The listing builds one solid part. Answer for the finished solid, in the listing's coordinates (mm). Give positions to 0.01 mm unless a question says otherwise; leave off trailing zeros. Answer as CSV lines item,"result". Start each with the question number.
(1) This flat-tipped pin is pushed along its axis until it touches: pin 1 Ø1.8 at (x, z) = (-119, -94) entering from +Y. Where does it stop, or does it pass through?
(2) Straight lines are drawn through the part: probe 1 along X at (y, z) = (1.9, -94); probe 2 along Z at (x, y) = (119, 1.9); probe 3 along Z at (x, y) = (-83, 2.9). For each, find the intervals that lie inside material, in ascending order.
(3) Find section A-A (y = 2.5). State how many separate pieces and enclosed holes the cut face has, then the cut area to 3 significant figures.
from build123d import *

# Parameters (mm, degrees)
SKETCH1_W           = 256
SKETCH1_H           = 206
BOSS_EXTRUDE1_DEPTH = 3
SKETCH2_R           = 1.5
CUT_EXTRUDE3_DEPTH  = 4
CUT_EXTRUDE6_DEPTH  = 4


with BuildPart() as part:
    # Sketch1 → Boss-Extrude1 (new body)
    with BuildSketch(Plane(origin=(0, 0, 0), x_dir=(1, 0, 0), z_dir=(0, 1, 0))):
        Rectangle(SKETCH1_W, SKETCH1_H)
    extrude(amount=BOSS_EXTRUDE1_DEPTH)

    # Sketch2 → Cut-Extrude3 (cut)
    with BuildSketch(Plane(origin=(0, 3, 0), x_dir=(1, 0, 0), z_dir=(0, 1, 0))):
        with Locations(Location((-119, 94, 0), (0, 0, 270))):
            Circle(SKETCH2_R)
        with Locations(Location((119, 94, 0), (0, 0, 270))):
            Circle(SKETCH2_R)
        with Locations(Location((119, -94, 0), (0, 0, 270))):
            Circle(SKETCH2_R)
        with Locations(Location((-119, -94, 0), (0, 0, 270))):
            Circle(SKETCH2_R)
    extrude(amount=-CUT_EXTRUDE3_DEPTH, mode=Mode.SUBTRACT)

    # Sketch5 → Cut-Extrude6 (cut)
    with BuildSketch(Plane(origin=(0, 3, 0), x_dir=(1, 0, 0), z_dir=(0, 1, 0))):
        with BuildLine():
            Line((-45.132956232, -35.122138654), (-33.270497542, -35.122138654))
            ThreePointArc((-33.270497542, -35.122138654), (-35.068849242, -42.49810977), (-39.012684657, -48.985418992))
            Line((-39.012684657, -48.985418992), (-47.527093129, -40.770618345))
            ThreePointArc((-47.527093129, -40.770618345), (-45.993141349, -38.089168216), (-45.132956232, -35.122138654))
        make_face()
        with BuildLine():
            Line((-34.575640496, -53.039857249), (-24.640816296, -63.279340889))
            ThreePointArc((-24.640816296, -63.279340889), (-16.366822155, -50.214880906), (-12.998109488, -35.122138654))
            Line((-12.998109488, -35.122138654), (-27.246251867, -35.122138654))
            ThreePointArc((-27.246251867, -35.122138654), (-29.467947906, -44.671268141), (-34.575640496, -53.039857249))
        make_face()
        with BuildLine():
            Line((-37.960142751, -56.424359504), (-27.720659111, -66.359183704))
            ThreePointArc((-27.720659111, -66.359183704), (-40.785119094, -74.633177845), (-55.877861346, -78.001890512))
            Line((-55.877861346, -78.001890512), (-55.877861346, -63.753748133))
            ThreePointArc((-55.877861346, -63.753748133), (-46.328731859, -61.532052094), (-37.960142751, -56.424359504))
        make_face()
        with BuildLine():
            Line((-55.877861346, -45.867043768), (-55.877861346, -57.729502458))
            ThreePointArc((-55.877861346, -57.729502458), (-48.50189023, -55.931150758), (-42.014581008, -51.987315343))
            Line((-42.014581008, -51.987315343), (-50.229381655, -43.472906871))
            ThreePointArc((-50.229381655, -43.472906871), (-52.910831784, -45.006858651), (-55.877861346, -45.867043768))
        make_face()
        with BuildLine():
            Line((-55.877861346, -2.246251867), (-55.877861346, 12.001890512))
            ThreePointArc((-55.877861346, 12.001890512), (-40.785119094, 8.633177845), (-27.720659111, 0.359183704))
            Line((-27.720659111, 0.359183704), (-37.960142751, -9.575640496))
            ThreePointArc((-37.960142751, -9.575640496), (-46.328731859, -4.467947906), (-55.877861346, -2.246251867))
        make_face()
        with BuildLine():
            Line((-55.877861346, -20.132956232), (-55.877861346, -8.270497542))
            ThreePointArc((-55.877861346, -8.270497542), (-48.50189023, -10.068849242), (-42.014581008, -14.012684657))
            Line((-42.014581008, -14.012684657), (-50.229381655, -22.527093129))
            ThreePointArc((-50.229381655, -22.527093129), (-52.910831784, -20.993141349), (-55.877861346, -20.132956232))
        make_face()
        with BuildLine():
            Line((-34.575640496, -12.960142751), (-24.640816296, -2.720659111))
            ThreePointArc((-24.640816296, -2.720659111), (-16.366822155, -15.785119094), (-12.998109488, -30.877861346))
            Line((-12.998109488, -30.877861346), (-27.246251867, -30.877861346))
            ThreePointArc((-27.246251867, -30.877861346), (-29.467947906, -21.328731859), (-34.575640496, -12.960142751))
        make_face()
        with BuildLine():
            Line((-45.132956232, -30.877861346), (-33.270497542, -30.877861346))
            ThreePointArc((-33.270497542, -30.877861346), (-35.068849242, -23.50189023), (-39.012684657, -17.014581008))
            Line((-39.012684657, -17.014581008), (-47.527093129, -25.229381655))
            ThreePointArc((-47.527093129, -25.229381655), (-45.993141349, -27.910831784), (-45.132956232, -30.877861346))
        make_face()
        with BuildLine():
            Line((-60.122138654, -45.867043768), (-60.122138654, -57.729502458))
            ThreePointArc((-60.122138654, -57.729502458), (-67.49810977, -55.931150758), (-73.985418992, -51.987315343))
            Line((-73.985418992, -51.987315343), (-65.770618345, -43.472906871))
            ThreePointArc((-65.770618345, -43.472906871), (-63.089168216, -45.006858651), (-60.122138654, -45.867043768))
        make_face()
        with BuildLine():
            Line((-60.122138654, -63.753748133), (-60.122138654, -78.001890512))
            ThreePointArc((-60.122138654, -78.001890512), (-75.214880906, -74.633177845), (-88.279340889, -66.359183704))
            Line((-88.279340889, -66.359183704), (-78.039857249, -56.424359504))
            ThreePointArc((-78.039857249, -56.424359504), (-69.671268141, -61.532052094), (-60.122138654, -63.753748133))
        make_face()
        with BuildLine():
            Line((-81.424359504, -53.039857249), (-91.359183704, -63.279340889))
            ThreePointArc((-91.359183704, -63.279340889), (-99.633177845, -50.214880906), (-103.001890512, -35.122138654))
            Line((-103.001890512, -35.122138654), (-88.753748133, -35.122138654))
            ThreePointArc((-88.753748133, -35.122138654), (-86.532052094, -44.671268141), (-81.424359504, -53.039857249))
        make_face()
        with BuildLine():
            Line((-70.867043768, -35.122138654), (-82.729502458, -35.122138654))
            ThreePointArc((-82.729502458, -35.122138654), (-80.931150758, -42.49810977), (-76.987315343, -48.985418992))
            Line((-76.987315343, -48.985418992), (-68.472906871, -40.770618345))
            ThreePointArc((-68.472906871, -40.770618345), (-70.006858651, -38.089168216), (-70.867043768, -35.122138654))
        make_face()
        with BuildLine():
            Line((-88.753748133, -30.877861346), (-103.001890512, -30.877861346))
            ThreePointArc((-103.001890512, -30.877861346), (-99.633177845, -15.785119094), (-91.359183704, -2.720659111))
            Line((-91.359183704, -2.720659111), (-81.424359504, -12.960142751))
            ThreePointArc((-81.424359504, -12.960142751), (-86.532052094, -21.328731859), (-88.753748133, -30.877861346))
        make_face()
        with BuildLine():
            Line((-70.867043768, -30.877861346), (-82.729502458, -30.877861346))
            ThreePointArc((-82.729502458, -30.877861346), (-80.931150758, -23.50189023), (-76.987315343, -17.014581008))
            Line((-76.987315343, -17.014581008), (-68.472906871, -25.229381655))
            ThreePointArc((-68.472906871, -25.229381655), (-70.006858651, -27.910831784), (-70.867043768, -30.877861346))
        make_face()
        with BuildLine():
            Line((-65.770618345, -22.527093129), (-73.985418992, -14.012684657))
            ThreePointArc((-73.985418992, -14.012684657), (-67.49810977, -10.068849242), (-60.122138654, -8.270497542))
            Line((-60.122138654, -8.270497542), (-60.122138654, -20.132956232))
            ThreePointArc((-60.122138654, -20.132956232), (-63.089168216, -20.993141349), (-65.770618345, -22.527093129))
        make_face()
        with BuildLine():
            Line((-78.039857249, -9.575640496), (-88.279340889, 0.359183704))
            ThreePointArc((-88.279340889, 0.359183704), (-75.214880906, 8.633177845), (-60.122138654, 12.001890512))
            Line((-60.122138654, 12.001890512), (-60.122138654, -2.246251867))
            ThreePointArc((-60.122138654, -2.246251867), (-69.671268141, -4.467947906), (-78.039857249, -9.575640496))
        make_face()
    extrude(amount=-CUT_EXTRUDE6_DEPTH, mode=Mode.SUBTRACT)


solid = part.part
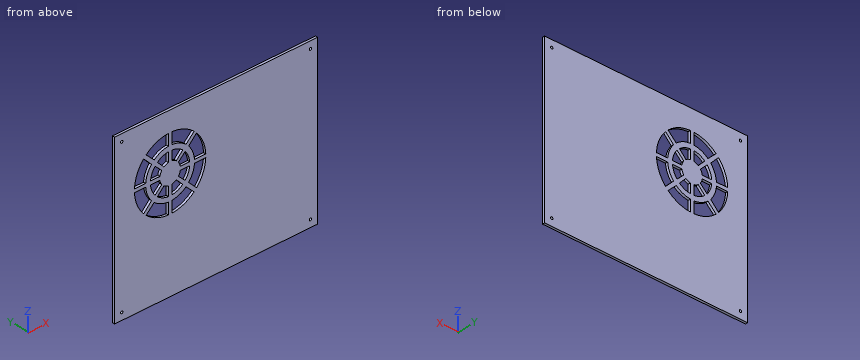
Result set:
1,pin 1,"through"
2,probe 1,"-128 to -120.5, -117.5 to 117.5, 120.5 to 128"
2,probe 2,"-103 to -95.5, -92.5 to 92.5, 95.5 to 103"
2,probe 3,"-103 to -4.48, 4.76 to 11.34, 14.96 to 51.04, 54.66 to 61.24, 70.48 to 103"
3,separate pieces,"1"
3,enclosed holes,"20"
3,area,"48,800 mm^2"
